from build123d import *

# Parameters (mm, degrees)
SKETCH1_R           = 16
BOSS_EXTRUDE1_DEPTH = 10
SKETCH2_R           = 18
SKETCH2_R_2         = 16
BOSS_EXTRUDE2_DEPTH = 2
SKETCH3_R           = 2
CUT_EXTRUDE1_DEPTH  = 10
SKETCH4_R           = 2
CUT_EXTRUDE2_DEPTH  = 10
CUT_EXTRUDE3_REACH  = 14
SKETCH5_R           = 3
FILLET1_R           = 5
BOSS_EXTRUDE4_START = -2
SKETCH8_R           = 16
SKETCH8_R_2         = 14
BOSS_EXTRUDE4_DEPTH = 2


with BuildPart() as part:
    # Sketch1 → Boss-Extrude1 (new body)
    with BuildSketch(Plane.XY):
        Polygon((-40, 83), (-70, 83), (-40, -7), (-40, -83), (40, -83), (40, -7), (10, 83), align=None)
        with Locations((-30, 60)):
            Circle(SKETCH1_R, mode=Mode.SUBTRACT)
    extrude(amount=BOSS_EXTRUDE1_DEPTH)

    # Sketch2 → Boss-Extrude2 (add)
    with BuildSketch(Plane.XY.offset(10)):
        with Locations((-30, 60)):
            Circle(SKETCH2_R)
        with Locations((-30, 60)):
            Circle(SKETCH2_R_2, mode=Mode.SUBTRACT)
    extrude(amount=BOSS_EXTRUDE2_DEPTH)

    # Sketch3 → Cut-Extrude1 (cut)
    with BuildSketch(Plane(origin=(0, 0, 0), x_dir=(-1, 0, 0), z_dir=(0, 0, -1))):
        with Locations((-15, -47)):
            Circle(SKETCH3_R)
        with Locations((25, -47)):
            Circle(SKETCH3_R)
    extrude(amount=-CUT_EXTRUDE1_DEPTH, mode=Mode.SUBTRACT)

    # Sketch4 → Cut-Extrude2 (cut)
    with BuildSketch(Plane(origin=(0, 0, 0), x_dir=(-1, 0, 0), z_dir=(0, 0, -1))):
        with Locations((5, -50)):
            Circle(SKETCH4_R)
    extrude(amount=-CUT_EXTRUDE2_DEPTH, mode=Mode.SUBTRACT)

    # Sketch5 → Cut-Extrude3 (cut, up to next)
    with BuildSketch(Plane(origin=(0, 0, 0), x_dir=(-1, 0, 0), z_dir=(0, 0, -1)), mode=Mode.PRIVATE) as cut_extrude3_sk1:
        with Locations((57, 76)):
            Circle(SKETCH5_R)
    cut_extrude3_tool1 = extrude(cut_extrude3_sk1.sketch, amount=-CUT_EXTRUDE3_REACH, mode=Mode.PRIVATE) & part.part
    add(cut_extrude3_tool1.solids().sort_by_distance((-57, 76, 0))[0], mode=Mode.SUBTRACT)

    # Fillet1
    fillet1_edges = [part.edges().sort_by_distance(p)[0] for p in [
        (-70, 83, 5),
        (10, 83, 5),
    ]]
    fillet(fillet1_edges, radius=FILLET1_R)

    # Sketch8 → Boss-Extrude4 (add)
    with BuildSketch(Plane(origin=(0, 0, 0), x_dir=(-1, 0, 0), z_dir=(0, 0, -1)).offset(BOSS_EXTRUDE4_START)):
        with Locations((30, 60)):
            Circle(SKETCH8_R)
        with Locations((30, 60)):
            Circle(SKETCH8_R_2, mode=Mode.SUBTRACT)
    extrude(amount=BOSS_EXTRUDE4_DEPTH)


solid = part.part
Verification items for the finished model (mm, model axes). A direction names the side the tool comes from. Coordinates: 2 decimals unless noted, no trailing zeros. Order: outer loops, then holes, each group sorted by start corner. A loop starts at its lowest first (then second) coordinate and runs counter-clockwise, first axis right, second up.
Item 1: Release check for a two-part mould opening along Y. For faces 1 (the face through (-5, -52, 5)), 2 (the face through (-42, 49, 12)), 3 (the face through (-54, 35, 5)) record: +Y half, -Y half, draft (parallel to the pull), parting line (faces both ways), or undercut.
Filled in:
face 1: undercut
face 2: draft
face 3: -Y half
Item 2: Section check A-A, the plane x = -30. Enter the section's corners in (y, z).
Filled in:
outline: (-83, 0) - (46, 0) - (46, 2) - (44, 2) - (44, 12) - (42, 12) - (42, 10) - (-83, 10) - close; (74, 0) - (83, 0) - (83, 10) - (78, 10) - (78, 12) - (76, 12) - (76, 2) - (74, 2) - close
Item 3: Section check C-C, the plane y = 52.5. Enter the section's corners in (x, z), then the cut area to 4 significant figures.
Filled in:
outline: (-59.83, 0) - (-41.82, 0) - (-41.82, 2) - (-44.13, 2) - (-44.13, 12) - (-46.36, 12) - (-46.36, 10) - (-59.83, 10) - close; (-18.18, 0) - (20.17, 0) - (20.17, 10) - (-13.64, 10) - (-13.64, 12) - (-15.87, 12) - (-15.87, 2) - (-18.18, 2) - close
area: 535.5 mm2
Item 4: Depth check by flat-ended pin: pin 1 (10 mm diameter, centred on x = -2.5, y = 21.5, fed in from -Z); pin 2 (3 mm diameter, centred on y = 51, z = 8, fed in from -X); pin 3 (6.5 mm diameter, centred on x = -25, y = -47, fed in from +Z). Enter the tip coordinate at first touch or a pass-through.
Filled in:
pin 1: stops at z = 0
pin 2: stops at x = -59.83
pin 3: stops at z = 10
Item 5: Material ranges on L1, parallel to Y at x = -30, z = 9.5; L2, parallel to Y at x = -25, z = 5; L3, parallel to Y at x = -26, z = 5.75, recorded low to high.
Filled in:
L1: y = -83 to 44, 76 to 83
L2: y = -83 to -49, -45 to 44.8, 75.2 to 83
L3: y = -83 to -48.73, -45.27 to 44.51, 75.49 to 83
Item 6: Access from +Z, -Z, +X, -X, +Y, -Y to the whole of each face (thin tool, end or side, straight path). Record for faces 4 (the face through (-29.93, 45.85, 2)), 5 (the face through (-40, -44, 5)), 6 (the face through (-25, -49, 5)).
Filled in:
face 4: +Z
face 5: +Z, -Z, -X, -Y
face 6: +Z, -Z
Item 7: Section check B-B, the plane z = 7.5. Enter the section's corners in (x, y), then the cut area to 3 significant figures.
Filled in:
outline: (-67.81, 76.42) - (-40, -7) - (-40, -83) - (40, -83) - (40, -7) - (11.14, 79.58) arc R5 ccw to (6.4, 83) - (-63.06, 83) arc R5 ccw to start; hole circle Ø6 at (-57, 76); hole circle Ø32 at (-30, 60); hole circle Ø4 at (-25, -47); hole circle Ø4 at (-5, -50); hole circle Ø4 at (15, -47)
area: 12,400 mm2
Item 8: Section check D-D, the plane x = 15. Enter the section's corners in (y, z), then the cut area to 3 significant figures.
Filled in:
outline: (-83, 0) - (-49, 0) - (-49, 10) - (-83, 10) - close; (-45, 0) - (68, 0) - (68, 10) - (-45, 10) - close
area: 1,470 mm2
